Geometry check sheet. Reference: the model listing, model coordinates, mm. Face numbers are marked on the shaded views. A direction names the side the tool comes from. Give positions to 0.01 mm unless a question says otherwise; leave off trailing zeros. Write each loop counter-clockwise with the first axis right and the second up, starting at its lowest first coordinate (ties: lowest second). Pieces come first, ordered by that corner, then holes. Notation, with made-up numbers: M -33.5,27.25 L -14.5,27.25 A19 cw -14.5,42.25 Z; hole C 32.5,79.5 d3. An arc over 180 degrees is marked long. One line per item, written item: value. Start each with the question number.
1. Cross-section at B-B on y = -4.5. Record the cut outline in (x, z), then the cut area to 3 significant figures.
2. Tool access check on the marked faces 1, 2 and 3. Record the directions out of +Z, -Z, +X, -X, +Y, -Y that give a thin tool (end or side, any length) a straight path to the whole face; none if there is none.
3. Release check for a two-part mould opening along X. For the marked faces 4, 5 and 6 record: pulls with the +X half, pulls with the -X half, needs draft (parallel to the pull), parting line crosses it, or undercut.
4. Gauge pin test, flat ends, axial feed: pin 1 (4 mm diameter, centred on x = -4.5, y = 7, fed in from +Z); pin 2 (0.9 mm diameter, centred on x = 0.5, y = -10, fed in from -Z); pin 3 (1 mm diameter, centred on y = 6, z = -7, fed in from +X). Record the tip position at first contact, or that the pin passes through.
5. Cross-section at A-A on x = 0. Record the cut outline in (y, z), then the cut area to 3 significant figures.
6. Scan lines: line 1 (X direction, y = -11, z = 0); line 2 (X direction, y = 2.5, z = 12.75); line 3 (Z direction, x = 10.5, y = 1). Record each from-to range of solid material in increasing order.
from build123d import *

# Parameters (mm, degrees)
SKETCH1_R           = 12.7
BOSS_EXTRUDE1_DEPTH = 10.16
BOSS_EXTRUDE2_START = -10.16
BOSS_EXTRUDE2_DEPTH = 10.16
CIRPATTERN1_COUNT   = 25
SKETCH3_R           = 6.35
BOSS_EXTRUDE3_DEPTH = 12.7
CUT_EXTRUDE1_DEPTH  = 6.35
FILLET1_R           = 1.27


with BuildPart() as part:
    # Sketch1 → Boss-Extrude1 (new body)
    with BuildSketch(Plane(origin=(0, 0, 0), x_dir=(1, 0, 0), z_dir=(0, 1, 0))):
        with Locations(Location((0, 0, 0), (0, 0, 270))):
            Circle(SKETCH1_R)
    extrude(amount=BOSS_EXTRUDE1_DEPTH)

    # Sketch2 → Boss-Extrude2 (add)
    with BuildSketch(Plane(origin=(0, 10.16, 0), x_dir=(1, 0, 0), z_dir=(0, 1, 0)).offset(BOSS_EXTRUDE2_START)):
        with BuildLine():
            Line((-0.745687793, 12.678089356), (-0.657137559, 13.690223169))
            Line((-0.657137559, 13.690223169), (-0.381, 13.943256622))
            Line((-0.381, 13.943256622), (0.381, 13.943256622))
            Line((0.381, 13.943256622), (0.657137559, 13.690223169))
            Line((0.657137559, 13.690223169), (0.745687793, 12.678089356))
            ThreePointArc((0.745687793, 12.678089356), (0, 12.7), (-0.745687793, 12.678089356))
        make_face()
    boss_extrude2 = extrude(amount=BOSS_EXTRUDE2_DEPTH)

    # CirPattern1: Boss-Extrude2 ×25 about axis
    cirpattern1_axis = Axis((0, 0, 0), (0, 1, 0))
    for i in range(1, CIRPATTERN1_COUNT):
        add(boss_extrude2.rotate(cirpattern1_axis, i * 360 / CIRPATTERN1_COUNT))

    # Sketch3 → Boss-Extrude3 (add)
    with BuildSketch(Plane.XZ):
        with Locations(Location((0, 0, 0), (0, 0, 90))):
            Circle(SKETCH3_R)
    extrude(amount=BOSS_EXTRUDE3_DEPTH)

    # Sketch4 → Cut-Extrude1 (cut)
    with BuildSketch(Plane.XZ.offset(12.7)):
        with BuildLine():
            Line((-1.425571464, 0.9525), (1.425571464, 0.9525))
            ThreePointArc((1.425571464, 0.9525), (0, -1.7145), (-1.425571464, 0.9525))
        make_face()
    extrude(amount=-CUT_EXTRUDE1_DEPTH, mode=Mode.SUBTRACT)

    # Fillet1
    fillet1_edges = [part.edges().sort_by_distance(p)[0] for p in [
        (0, 0, -6.35),
    ]]
    fillet(fillet1_edges, radius=FILLET1_R)


solid = part.part
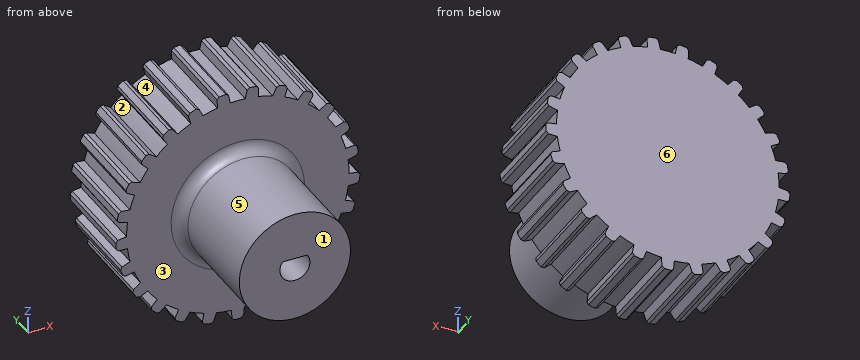
Report:
1. outline: C 0,0 d12.7
1. area: 127 mm^2
2. face 1: +Z, -Z, +X, -X, -Y
2. face 2: +Y, -Y
2. face 3: -Y
3. face 4: undercut
3. face 5: parting line crosses it
3. face 6: needs draft
4. pin 1: stops at z = 13.1
4. pin 2: stops at z = -6.35
4. pin 3: stops at x = 11.98
5. outline: M -12.7,-6.35 L -1.27,-6.35 A1.27 cw 0,-7.62 L 0,-13.94 L 10.16,-13.94 L 10.16,12.7 L 0,12.7 L 0,7.62 A1.27 cw -1.27,6.35 L -12.7,6.35 L -12.7,0.95 L -6.35,0.95 L -6.35,-1.71 L -12.7,-1.71 Z
5. area: 416 mm^2
6. line 1: x = -6.35 to -1.71, 1.71 to 6.35
6. line 2: x = -5.52 to -4.32, -2.34 to -0.87, 0.87 to 2.34, 4.32 to 5.52
6. line 3: z = -7.52 to 7.14, 7.76 to 9.18
